Build history of the part. All positions in model axes, mm. A direction names the side the tool comes from. Coordinates: 2 decimals unless noted, no trailing zeros. Order: outer loops, then holes, each group sorted by start corner. A loop starts at its lowest first (then second) coordinate and runs counter-clockwise, first axis right, second up. Notation, with made-up numbers: (82, 38) - (112, 38) arc R28 cw to (112, 67) - close; hole circle Ø3 at (-15.5, 31). An arc over 180 degrees is marked (long way). Write each question's results on one line, items separated by ' | '.
from build123d import *

# Parameters (mm, degrees)
SKETCH1_W            = 150
SKETCH1_H            = 80
SKETCH1_W_2          = 10
SKETCH1_H_2          = 20
BOSS_EXTRUDE1_DEPTH  = 10
FILLET1_R            = 2
FILLET2_R            = 5
BOSS_EXTRUDE2_DEPTH  = 23
SKETCH2_3_W          = 34.5
SKETCH2_3_H          = 20.5
CUT_EXTRUDE1_DEPTH   = 10
SKETCH3_W            = 5
SKETCH3_H            = 20.5
SKETCH3_R            = 1.1
BOSS_EXTRUDE3_DEPTH  = 3
CUT_EXTRUDE2_REACH   = 101.569
SKETCH7_W            = 5
SKETCH7_H            = 20.5
CUT_EXTRUDE3_DEPTH   = 1
SKETCH14_W           = 23
SKETCH14_H           = 11
CUT_EXTRUDE4_DEPTH   = 6
FILLET4_R            = 1
SKETCH15_R           = 3.25
CUT_EXTRUDE5_DEPTH   = 10
BOSS_EXTRUDE8_DEPTH  = 15
SKETCH16_3_W         = 19
SKETCH16_3_H         = 5
BOSS_EXTRUDE9_DEPTH  = 5
SKETCH17_R           = 1.7
CUT_EXTRUDE6_DEPTH   = 4
FILLET10_R           = 2
FILLET11_R           = 2
SKETCH18_W           = 67.5
SKETCH18_H           = 65
CUT_EXTRUDE7_DEPTH   = 89.056799851
SKETCH20_W           = 3
SKETCH20_H           = 50
BOSS_EXTRUDE11_DEPTH = 10
FILLET13_R           = 1
FILLET14_R           = 1
CUT_EXTRUDE8_REACH   = 160.71
SKETCH21_W           = 10
SKETCH21_H           = 30
FILLET15_R           = 1
SKETCH22_W           = 30
SKETCH22_H           = 3
SKETCH22_W_2         = 12
BOSS_EXTRUDE12_DEPTH = 10
FILLET16_R           = 1
FILLET17_R           = 1
FILLET18_R           = 2


with BuildPart() as part:
    # Sketch1 → Boss-Extrude1 (new body)
    with BuildSketch(Plane.XY):
        Rectangle(SKETCH1_W, SKETCH1_H)
        with Locations((-15, 0)):
            Rectangle(SKETCH1_W_2, SKETCH1_H_2, mode=Mode.SUBTRACT)
    extrude(amount=BOSS_EXTRUDE1_DEPTH)

    # Fillet1
    fillet1_edges = [part.edges().sort_by_distance(p)[0] for p in [
        (-10, -10, 5),
        (-10, 10, 5),
        (-20, 10, 5),
        (-20, -10, 5),
    ]]
    fillet(fillet1_edges, radius=FILLET1_R)

    # Fillet2
    fillet2_edges = [part.edges().sort_by_distance(p)[0] for p in [
        (75, -40, 5),
        (-75, -40, 5),
        (-75, 40, 5),
        (75, 40, 5),
    ]]
    fillet(fillet2_edges, radius=FILLET2_R)

    # Sketch2 → Boss-Extrude2 (add)
    with BuildSketch(Plane.XY.offset(10)):
        Polygon((57, 10.25), (57, -10.25), (22.5, -10.25), (11, -10.25), (11, -21.25), (68.5, -21.25), (68.5, 21.25), (11, 21.25), (11, 10.25), (22.5, 10.25), align=None)
    extrude(amount=BOSS_EXTRUDE2_DEPTH)

    # Sketch2<3> → Cut-Extrude1 (cut)
    with BuildSketch(Plane.XY.offset(10)):
        with Locations((39.75, 0)):
            Rectangle(SKETCH2_3_W, SKETCH2_3_H)
    extrude(amount=-CUT_EXTRUDE1_DEPTH, mode=Mode.SUBTRACT)

    # Sketch3 → Boss-Extrude3 (add)
    # profile 1 of 2: a face of its own
    with BuildSketch(Plane.XY.offset(10)):
        with Locations((25, 0)):
            Rectangle(SKETCH3_W, SKETCH3_H)
        with Locations((24.75, 8)):
            Circle(SKETCH3_R, mode=Mode.SUBTRACT)
        with Locations((24.75, -8)):
            Circle(SKETCH3_R, mode=Mode.SUBTRACT)
    # profile 2 of 2: a face of its own
    with BuildSketch(Plane.XY.offset(10)):
        with Locations((54.5, 0)):
            Rectangle(SKETCH3_W, SKETCH3_H)
        with Locations((54.75, 8)):
            Circle(SKETCH3_R, mode=Mode.SUBTRACT)
        with Locations((54.75, -8)):
            Circle(SKETCH3_R, mode=Mode.SUBTRACT)
    extrude(amount=-BOSS_EXTRUDE3_DEPTH)

    # Sketch4 → Cut-Loft2 section 0
    with BuildSketch(Plane(origin=(0, 0, 7), x_dir=(-1, 0, 0), z_dir=(0, 0, -1))):
        with BuildLine():
            Line((-22.5, 10.25), (-57, 10.25))
            Line((-57, 10.25), (-57, -10.25))
            Line((-57, -10.25), (-22.5, -10.25))
            Line((-22.5, -10.25), (-22.5, 10.25))
        make_face()
    # Sketch5 → Cut-Loft2 section 1
    with BuildSketch(Plane(origin=(0, 0, 0), x_dir=(-1, 0, 0), z_dir=(0, 0, -1))):
        with BuildLine():
            Line((-67, -18.25), (-12.5, -18.25))
            Line((-12.5, -18.25), (-12.5, 18.25))
            Line((-12.5, 18.25), (-67, 18.25))
            Line((-67, 18.25), (-67, -18.25))
        make_face()
    loft(mode=Mode.SUBTRACT)

    # Cut-Extrude2: up to this plane
    cut_extrude2_end = Plane(origin=(4.110738255, 0, -5.872483221), z_dir=(-0.5734623443633287, 0, 0.8192319205190403))
    # Sketch6 → Cut-Extrude2 (cut, up to the surface)
    with BuildSketch(Plane.ZY.offset(10), mode=Mode.PRIVATE) as cut_extrude2_sk1:
        with BuildLine():
            Line((0, 6), (0, -6))
            ThreePointArc((0, -6), (6, 0), (0, 6))
        make_face()
    cut_extrude2_tool1 = split(extrude(cut_extrude2_sk1.sketch, amount=-CUT_EXTRUDE2_REACH, mode=Mode.PRIVATE), bisect_by=cut_extrude2_end, keep=Keep.BOTH, mode=Mode.PRIVATE)
    add(cut_extrude2_tool1.solids().sort_by_distance((-10, 0, 2.546479))[0], mode=Mode.SUBTRACT)

    # Sketch7 → Cut-Extrude3 (cut)
    with BuildSketch(Plane(origin=(0, 0, 7), x_dir=(-1, 0, 0), z_dir=(0, 0, -1))):
        with Locations((-54.5, 0)):
            Rectangle(SKETCH7_W, SKETCH7_H)
        with Locations((-25, 0)):
            Rectangle(SKETCH7_W, SKETCH7_H)
    extrude(amount=-CUT_EXTRUDE3_DEPTH, mode=Mode.SUBTRACT)

    # Sketch14 → Cut-Extrude4 (cut)
    with BuildSketch(Plane.ZY.offset(-11)):
        with Locations((21.5, -15.75)):
            Rectangle(SKETCH14_W, SKETCH14_H)
        with Locations((21.5, 15.75)):
            Rectangle(SKETCH14_W, SKETCH14_H)
    extrude(amount=-CUT_EXTRUDE4_DEPTH, mode=Mode.SUBTRACT)

    # Fillet4
    fillet4_edges = [part.edges().sort_by_distance(p)[0] for p in [
        (52, 10.25, 9),
        (52, -10.25, 9),
        (27.5, -10.25, 9),
        (27.5, 10.25, 9),
    ]]
    fillet(fillet4_edges, radius=FILLET4_R)

    # Sketch15 → Cut-Extrude5 (cut)
    with BuildSketch(Plane.XY.offset(10)):
        with Locations((-67.5, 32.5)):
            Circle(SKETCH15_R)
        with Locations((0, 32.5)):
            Circle(SKETCH15_R)
        with Locations((67.5, 32.5)):
            Circle(SKETCH15_R)
        with Locations((67.5, -32.5)):
            Circle(SKETCH15_R)
        with Locations((0, -32.5)):
            Circle(SKETCH15_R)
        with Locations((-67.5, -32.5)):
            Circle(SKETCH15_R)
    extrude(amount=-CUT_EXTRUDE5_DEPTH, mode=Mode.SUBTRACT)

    # Sketch16 → Boss-Extrude8 (add)
    with BuildSketch(Plane.XY.offset(10)):
        Polygon((-49, -24.05), (-49, 24.05), (-30, 24.05), (-30, -24.05), (-30, -29.05), (-25, -29.05), (-25, 29.05), (-54, 29.05), (-54, -29.05), (-49, -29.05), align=None)
    extrude(amount=BOSS_EXTRUDE8_DEPTH)

    # Sketch16<3> → Boss-Extrude9 (add)
    with BuildSketch(Plane.XY.offset(10)):
        with Locations((-39.5, -26.55)):
            Rectangle(SKETCH16_3_W, SKETCH16_3_H)
    extrude(amount=BOSS_EXTRUDE9_DEPTH)

    # Sketch17 → Cut-Extrude6 (cut)
    with BuildSketch(Plane.XY.offset(25)):
        with Locations((-27.5, 3.05)):
            Circle(SKETCH17_R)
        with Locations((-51.5, -6.95)):
            Circle(SKETCH17_R)
    extrude(amount=-CUT_EXTRUDE6_DEPTH, mode=Mode.SUBTRACT)

    # Fillet10
    fillet10_edges = [part.edges().sort_by_distance(p)[0] for p in [
        (-30, -26.55, 15),
        (-49, -26.55, 15),
    ]]
    fillet(fillet10_edges, radius=FILLET10_R)

    # Fillet11
    fillet11_edges = [part.edges().sort_by_distance(p)[0] for p in [
        (-39.5, -29.05, 10),
        (-25, -29.05, 17.5),
        (-25, 29.05, 17.5),
        (-54, 0, 10),
        (-54, 29.05, 17.5),
        (-54, -29.05, 17.5),
        (-39.5, 29.05, 10),
        (-25, 0, 10),
    ]]
    fillet(fillet11_edges, radius=FILLET11_R)

    # Sketch18 → Cut-Extrude7 (cut, through all)
    with BuildSketch(Plane.XY.offset(10)):
        with Locations((-33.75, 0)):
            Rectangle(SKETCH18_W, SKETCH18_H)
    extrude(amount=CUT_EXTRUDE7_DEPTH, mode=Mode.SUBTRACT)

    # Sketch20 → Boss-Extrude11 (add)
    with BuildSketch(Plane.XY.offset(10)):
        with Locations((-73.5, 0)):
            Rectangle(SKETCH20_W, SKETCH20_H)
        with Locations((-21.5, 0)):
            Rectangle(SKETCH20_W, SKETCH20_H)
    extrude(amount=BOSS_EXTRUDE11_DEPTH)

    # Fillet13
    fillet13_edges = [part.edges().sort_by_distance(p)[0] for p in [
        (-75, 25, 15),
        (-75, -25, 15),
        (-72, -25, 15),
        (-72, 25, 15),
    ]]
    fillet(fillet13_edges, radius=FILLET13_R)

    # Fillet14
    fillet14_edges = [part.edges().sort_by_distance(p)[0] for p in [
        (-23, 25, 15),
        (-23, -25, 15),
        (-20, -25, 15),
        (-20, 25, 15),
    ]]
    fillet(fillet14_edges, radius=FILLET14_R)

    # Sketch21 → Cut-Extrude8 (cut, up to next)
    with BuildSketch(Plane.ZY.offset(75), mode=Mode.PRIVATE) as cut_extrude8_sk1:
        with Locations((15, 19)):
            Rectangle(SKETCH21_W, SKETCH21_H)
    cut_extrude8_tool1 = extrude(cut_extrude8_sk1.sketch, amount=-CUT_EXTRUDE8_REACH, mode=Mode.PRIVATE) & part.part
    add(cut_extrude8_tool1.solids().sort_by_distance((-75, 19, 15))[0], mode=Mode.SUBTRACT)

    # Fillet15
    fillet15_edges = [part.edges().sort_by_distance(p)[0] for p in [
        (-75, 4, 15),
        (-72, 4, 15),
    ]]
    fillet(fillet15_edges, radius=FILLET15_R)

    # Sketch22 → Boss-Extrude12 (add)
    with BuildSketch(Plane.XY.offset(10)):
        with Locations((-47.5, 30.2)):
            Rectangle(SKETCH22_W, SKETCH22_H)
        with Locations((-32, -30.2)):
            Rectangle(SKETCH22_W_2, SKETCH22_H)
    extrude(amount=BOSS_EXTRUDE12_DEPTH)

    # Fillet16
    fillet16_edges = [part.edges().sort_by_distance(p)[0] for p in [
        (-62.5, 31.7, 15),
        (-62.5, 28.7, 15),
        (-32.5, 28.7, 15),
        (-32.5, 31.7, 15),
    ]]
    fillet(fillet16_edges, radius=FILLET16_R)

    # Fillet17
    fillet17_edges = [part.edges().sort_by_distance(p)[0] for p in [
        (-38, -28.7, 15),
        (-38, -31.7, 15),
        (-26, -31.7, 15),
        (-26, -28.7, 15),
    ]]
    fillet(fillet17_edges, radius=FILLET17_R)

    # Fillet18
    fillet18_edges = [part.edges().sort_by_distance(p)[0] for p in [
        (17, -10.25, 21.5),
        (17, -21.25, 21.5),
        (17, 21.25, 21.5),
        (17, 10.25, 21.5),
        (68.5, -21.25, 21.5),
        (68.5, 21.25, 21.5),
    ]]
    fillet(fillet18_edges, radius=FILLET18_R)


solid = part.part
1. Band-saw the part on A-A on x = 0. Give the cut face in (y, z).
Solved:
outline: (-40, 0) - (-35.75, 0) - (-35.75, 10) - (-40, 10) - close; (-29.25, 0) - (-6, 0) arc R6 cw to (6, 0) - (29.25, 0) - (29.25, 10) - (-29.25, 10) - close; (35.75, 0) - (40, 0) - (40, 10) - (35.75, 10) - close
2. Two-plate mould, pull along Y, no slides. Class faces 4 (the face through (-0.705, 29.327, 5.07)), 5 (the face through (-20, 0, 12)), 6 (the face through (75, 0, 5)), 7 (the face through (43, 21.25, 21)): +Y half, -Y half, draft (parallel to the pull), parting line (faces both ways), or undercut.
Solved:
face 4: undercut | face 5: undercut | face 6: draft | face 7: +Y half
3. Tool access for faces 1 (the face through (68.5, 0, 21)), 2 (the face through (-32, -28.7, 15)), 3 (the face through (-23, 0, 15)): list every direction of +Z, -Z, +X, -X, +Y, -Y with a clear straight run to the whole face (end or side of a thin tool).
Solved:
face 1: +Z, +X, +Y, -Y | face 2: +Z, +X, -X | face 3: +Z, +Y, -Y
4. Band-saw the part on C-C on x = -67.5. Give the cut face in (y, z), then the cut area to 3 significant figures.
Solved:
outline: (-40, 0) - (-35.75, 0) - (-35.75, 10) - (-40, 10) - close; (-29.25, 0) - (29.25, 0) - (29.25, 10) - (-29.25, 10) - close; (35.75, 0) - (40, 0) - (40, 10) - (35.75, 10) - close | area: 670 mm2
5. Band-saw the part on B-B on x = -42. Give the cut face in (y, z).
Solved:
outline: (-40, 0) - (40, 0) - (40, 10) - (31.7, 10) - (31.7, 20) - (28.7, 20) - (28.7, 10) - (-40, 10) - close
6. Band-saw the part on D-D on z = 4.5. Give the number of separate pieces and of enclosed holes in the cut face, then the cut area to 3 significant figures.
Solved:
separate pieces: 1 | enclosed holes: 7 | area: 10,300 mm2
7. Probe line 1 (Y direction, x = 54.75, z = 9.55); line 2 (X direction, y = -17, z = 12); line 3 (X direction, y = -31, z = 1.5). List the from-to ranges inside material, lowest first.
Solved:
line 1: y = -40 to -9.1, -6.9 to 6.9, 9.1 to 40 | line 2: x = -75 to -72, -23 to -20, 17 to 68.5 | line 3: x = -75 to -70.38, -64.62 to -2.88, 2.88 to 64.62, 70.38 to 75
8. Drop flat-ended pins along their axis: pin 1 Ø10 at (y, z) = (-0.5, 14) entering from +X; pin 2 Ø5.5 at (y, z) = (15, 19.5) entering from -X; pin 3 Ø6 at (x, z) = (38, 27.5) entering from -Y; pin 4 Ø2.5 at (x, y) = (24.75, -8) entering from -Z. Give the stop position or say it passes through.
Solved:
pin 1: stops at x = 75 | pin 2: stops at x = -23 | pin 3: stops at y = -21.25 | pin 4: stops at z = 8
